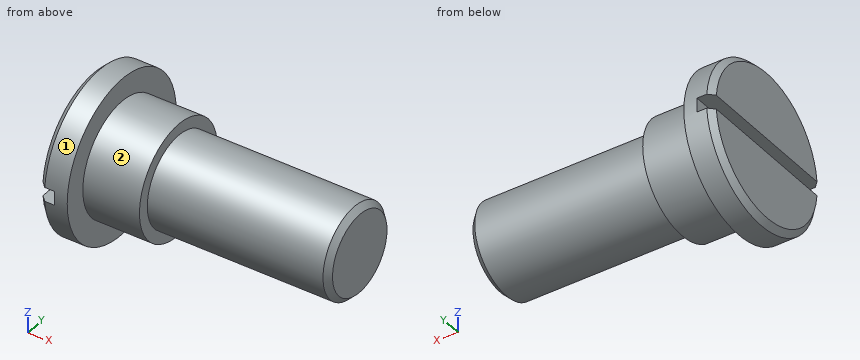
from build123d import *

# Parameters (mm, degrees)
F0_R          = 8
F1_DEPTH      = 42
F1_DEPTH_BACK = 5
F0_R_2        = 10
F2_DEPTH      = 10
F2_DEPTH_BACK = 5
F0_R_3        = 14
F3_DEPTH      = 5
F4_SIZE       = 1
F5_W          = 58
F5_H          = 2.5
F6_DEPTH      = 25
F6_DEPTH_BACK = 25


with BuildPart() as f1:
    # F0 (on Right) → F1 (new body, two sides)
    with BuildSketch(Plane.YZ) as f1_sk:
        Circle(F0_R)
    extrude(amount=F1_DEPTH)
    extrude(f1_sk.sketch, amount=-F1_DEPTH_BACK)

    # F0 (on Right) → F2 (join, two sides)
    with BuildSketch(Plane.YZ) as f2_sk:
        Circle(F0_R_2)
        Circle(F0_R, mode=Mode.SUBTRACT)
    extrude(amount=F2_DEPTH)
    extrude(f2_sk.sketch, amount=-F2_DEPTH_BACK)

    # F0 (on Right) → F3 (join)
    with BuildSketch(Plane.YZ):
        Circle(F0_R_3)
        Circle(F0_R_2, mode=Mode.SUBTRACT)
    extrude(amount=-F3_DEPTH)

    # F4
    f4_edges = [f1.edges().sort_by_distance(p)[0] for p in [
        (-5, -14, 0),
        (42, -8, 0),
    ]]
    chamfer(f4_edges, length=F4_SIZE)

    # F5 (on Front) → F6 (cut, two sides)
    with BuildSketch(Plane.XZ) as f6_sk:
        with Locations((-31.278737, 0)):
            Rectangle(F5_W, F5_H)
    extrude(amount=F6_DEPTH, mode=Mode.SUBTRACT)
    extrude(f6_sk.sketch, amount=-F6_DEPTH_BACK, mode=Mode.SUBTRACT)


solid = f1.part
Read the model definition and answer for the solid it produces. Units are mm, in the model's axes. Face numbers are marked on the shaded views. A direction names the side the tool comes from. Coordinates: 2 decimals unless noted, no trailing zeros. Order: outer loops, then holes, each group sorted by start corner. A loop starts at its lowest first (then second) coordinate and runs counter-clockwise, first axis right, second up. Notation, with made-up numbers: (-3, 20) -> (33, 20) arc R17 cw to (33, 39) -> close; hole circle Ø11 at (30.25, 49). An arc over 180 degrees is marked (long way). Answer as a JSON object with one key per item and string values.
1) A tool of negligible diameter and unlimited length cuts with its end or side. For the marked faces 1 and 2, from which of +Z, -Z, +X, -X, +Y, -Y can it reach the whole face along a straight path? Write none if from no direction.
Model answer:
{"face 1": "+X, -X", "face 2": "+X"}
2) Consider line 1 along X through (y, z) = (-6.25, -8.75); line 2 along Z through (x, y) = (15, 0); line 3 along X through (y, z) = (-7.5, 6.25). Determine where each line is inside the solid, lowest interval first. Write a range as from..to.
Model answer:
{"line 1": "x = -5..0", "line 2": "z = -8..8", "line 3": "x = -5..10"}
3) A cutting plane is placed at D-D, the plane x = 38. Determine the outline of the cut face in (y, z), plus the area to 3 significant figures.
Model answer:
{"outline": "circle Ø16 at (0, 0)", "area": "201 mm²"}
4) Each of these flat-tipped pins is pushed along its axis until it touches: pin 1 (6 mm diameter, centred on y = -2.5, z = 7.5, fed in from +X); pin 2 (2 mm diameter, centred on x = -3, y = 2.5, fed in from -Z); pin 3 (1 mm diameter, centred on x = 15, z = 6, fed in from -Y); pin 4 (0.8 mm diameter, centred on x = -4, y = -5, fed in from +Z). Where does it stop, or does it pass through?
Model answer:
{"pin 1": "stops at x = 42", "pin 2": "stops at z = -13.92", "pin 3": "stops at y = -5.81", "pin 4": "stops at z = 13.22"}
5) A cutting plane is placed at B-B, the plane y = 0. Determine the outline of the cut face in (x, z).
Model answer:
{"outline": "(-5, -13) -> (-4, -14) -> (0, -14) -> (0, -10) -> (10, -10) -> (10, -8) -> (41, -8) -> (42, -7) -> (42, 7) -> (41, 8) -> (10, 8) -> (10, 10) -> (0, 10) -> (0, 14) -> (-4, 14) -> (-5, 13) -> (-5, 1.25) -> (-2.28, 1.25) -> (-2.28, -1.25) -> (-5, -1.25) -> close"}
6) A cutting plane is placed at C-C, the plane x = 8. Determine the outline of the cut face in (y, z).
Model answer:
{"outline": "circle Ø20 at (0, 0)"}
7) A cutting plane is placed at A-A, the plane z = 0. Determine the outline of the cut face in (x, y).
Model answer:
{"outline": "(-2.28, -14) -> (0, -14) -> (0, -10) -> (10, -10) -> (10, -8) -> (41, -8) -> (42, -7) -> (42, 7) -> (41, 8) -> (10, 8) -> (10, 10) -> (0, 10) -> (0, 14) -> (-2.28, 14) -> close"}
